Autodesk Inventor part; units mm, degrees
ref_plane "YZ Plane" through (0, 0, 0) normal (1, 0, 0) x (0, 1, 0)
ref_plane "XZ Plane" through (0, 0, 0) normal (0, 1, 0) x (-1, 0, 0)
ref_plane "XY Plane" through (0, 0, 0) normal (0, 0, 1) x (1, 0, 0)
sketch "Sketch1" plane through (0, 0, 0) normal (0, 1, 0) x (-1, 0, 0)
  arc A0 (5.5, -5.5) -> (11, 0) centre (5.5, 0) ccw
  line L0 (3.2, -5.5) -> (3.2, -10.5)
  line L1 (3.2, -10.5) -> (0, -10.5)
  line L2 (0, -10.5) -> (0, 10.5)
  line L3 (0, 10.5) -> (3.2, 10.5)
  line L4 (3.2, 10.5) -> (3.2, 5.5)
  arc A1 (11, 0) -> (5.5, 5.5) centre (5.5, 0) ccw
  line L5 (3.2, 5.5) -> (11, 0) construction
  line L6 (3.2, -5.5) -> (11, 0) construction
  line L7 (5.5, 5.5) -> (3.2, 5.5)
  line L8 (3.2, -5.5) -> (5.5, -5.5)
  point P0 (0, 0)
  point P1 (0, 0)
  dimension "d0" = 3.2
  dimension "d1" = 21
  dimension "d6" = 11
  dimension "d21" = 11
extrude "Extrusion1" add sketch "Sketch1" along normal blind 21
sketch "Sketch2" plane through (0, 0, 10.5) normal (1, 0, 0) x (0, 0, -1)
  circle A0 centre (18.45, 17.65) radius 1.2
  circle A1 centre (2.55, 3.35) radius 1.2
  line L0 (18.45, 17.65) -> (18.45, 3.35) construction
  line L1 (18.45, 3.35) -> (2.55, 3.35) construction
  line L2 (21, 0) -> (21, 21)
  line L3 (0, 0) -> (0, 21)
  line L4 (18.45, 17.65) -> (21, 17.65) construction
  line L5 (18.45, 17.65) -> (21, 21) construction
  line L6 (0, 0) -> (2.55, 3.35) construction
  line L7 (2.55, 3.35) -> (0, 3.35) construction
  line L8 (21, 14.3) -> (16.55, 14.3)
  line L9 (16.55, 14.3) -> (16.55, 0)
  line L10 (16.55, 0) -> (21, 0)
  line L11 (0, 6.7) -> (4.45, 6.7)
  line L12 (4.45, 6.7) -> (4.45, 21)
  line L13 (4.45, 21) -> (0, 21)
  line L14 (21, 14.3) -> (18.45, 17.65) construction
  point P0 (10.5, 0)
  dimension "d9" = 15.9
  dimension "d10" = 14.3
  dimension "d11" = 2.4
  dimension "d12" = 1.9
extrude "Extrusion2" cut sketch "Sketch2" against normal up to surface (3.2 mm away)
sketch "Sketch3" plane through (0, 0, 0) normal (0, -1, 0) x (1, 0, 0)
  arc A0 (-3.2, 5.5) -> (-3.2, -5.5) centre (-5.5, 0) ccw
  circle A1 centre (-5.5, 0) radius 1.5875
  point P0 (0, 0)
  dimension "d15" = 3.175
extrude "Extrusion3" add sketch "Sketch3" along normal blind 8
sketch "Sketch4" plane through (0, 21, 0) normal (0, 1, 0) x (1, 0, 0)
  arc A0 (-3.2, 5.5) -> (-3.2, -5.5) centre (-5.5, 0) ccw construction
  circle A1 centre (-5.5, 0) radius 1.5875
  point P0 (0, 0)
  dimension "d18" = 3.175
extrude "Extrusion4" add sketch "Sketch4" along normal blind 8
properties part number "Power Resistor - HSA25" material "Gold"
Check sheet for the modelled part. Datum: model origin and axes. Units: mm. A direction names the side the tool comes from. Coordinates: 2 decimals unless noted, no trailing zeros. Loops run counter-clockwise (first coordinate to the right, second up) from the corner with the lowest first, then second, coordinate; pieces in that order, holes last. Notation, with made-up numbers: (-36, 14) -> (0, 14) arc R35 ccw to (0, 48) -> close; hole circle Ø8 at (-37.5, 50.25). An arc over 180 degrees is marked (long way). Answer in a Markdown table with one row per item.
1. Release check for a two-part mould opening along Y. For faces 4 (the face through (-6.76, 24.944, -0.966)), 5 (the face through (-1.58, 2.89, 6.84)), 6 (the face through (-4, 0, 2)) record: released by +Y, released by -Y, zero draft, split by the parting line, or undercut.
Check values:
| item | result |
|---|---|
| face 4 | zero draft |
| face 5 | undercut |
| face 6 | released by -Y |
2. Sectioned sample at A-A, the plane z = -7.95. Record the boundary of the cut face in (x, y), then the cut area to 3 significant figures.
Check values:
| item | result |
|---|---|
| outline | (-3.2, 14.3) -> (0, 14.3) -> (0, 16.45) -> (-3.2, 16.45) -> close; (-3.2, 18.85) -> (0, 18.85) -> (0, 21) -> (-3.2, 21) -> close |
| area | 13.8 mm2 |
3. Sectioned sample at C-C, the plane y = 17.65. Record the boundary of the cut face in (x, z), then the cut area to 3 significant figures.
Check values:
| item | result |
|---|---|
| outline | (-5.5, -5.5) -> (-3.2, -5.5) -> (-3.2, -6.75) -> (0, -6.75) -> (0, 6.05) -> (-3.2, 6.05) -> (-3.2, 5.5) -> (-5.5, 5.5) arc R5.5 ccw to start; (-3.2, -10.5) -> (0, -10.5) -> (0, -9.15) -> (-3.2, -9.15) -> close |
| area | 118 mm2 |
4. Go/stop test with flat-tipped pins: pin 1 (3.5 mm diameter, centred on x = -1, y = 7, fed in from -Z); pin 2 (3.5 mm diameter, centred on x = -5.5, z = -4.5, fed in from +Y); pin 3 (2.5 mm diameter, centred on x = -1, y = 15.5, fed in from +Z). Record where each tip stops, or that it passes through.
Check values:
| item | result |
|---|---|
| pin 1 | stops at z = -6.05 |
| pin 2 | stops at y = 21 |
| pin 3 | stops at z = 6.05 |
5. Sectioned sample at D-D, the plane z = 0. Record the boundary of the cut face in (x, y), then the cut area to 3 significant figures.
Check values:
| item | result |
|---|---|
| outline | (-11, 0) -> (-7.09, 0) -> (-7.09, -8) -> (-3.91, -8) -> (-3.91, 0) -> (0, 0) -> (0, 21) -> (-3.91, 21) -> (-3.91, 29) -> (-7.09, 29) -> (-7.09, 21) -> (-11, 21) -> close |
| area | 282 mm2 |
6. Material ranges on line 1 along Y through (x, z) = (-1.55, 7.95); line 2 along Y through (x, z) = (-2.2, -7.95); line 3 along Y through (x, z) = (-3.5, -3.5), recorded low to high. Write a range as [from, to].
Check values:
| item | result |
|---|---|
| line 1 | y = [0, 2.15], [4.55, 6.7] |
| line 2 | y = [14.3, 16.45], [18.85, 21] |
| line 3 | y = [0, 21] |
7. Sectioned sample at B-B, the plane x = -2.75. Record the boundary of the cut face in (y, z), then the cut area to 3 significant figures.
Check values:
| item | result |
|---|---|
| outline | (0, -6.05) -> (14.3, -6.05) -> (14.3, -10.5) -> (21, -10.5) -> (21, 6.05) -> (6.7, 6.05) -> (6.7, 10.5) -> (0, 10.5) -> close; hole circle Ø2.4 at (3.35, 7.95); hole circle Ø2.4 at (17.65, -7.95) |
| area | 305 mm2 |
8. Access from +Z, -Z, +X, -X, +Y, -Y to the whole of each face (thin tool, end or side, straight path). Record for faces 1 (the face through (-2, 14, 6.05)), 2 (the face through (-6.76, -3.944, 0.966)), 3 (the face through (-4, 10, -5.5)).
Check values:
| item | result |
|---|---|
| face 1 | +Z, +X, -X, +Y |
| face 2 | -Y |
| face 3 | -Z, -X, +Y, -Y |
